Source: three-view drawing plus pictorial views. Frame: mm from the lowest corner of the part. A direction names the side the tool comes from. Coordinates: 2 decimals unless noted, no trailing zeros. Loops run counter-clockwise (first coordinate to the right, second up) from the corner with the lowest first, then second, coordinate; pieces in that order, holes last. Notation, with made-up numbers: (-29, -34.5) - (22, -34.5) arc R23 ccw to (22, -4.5) - close; hole circle Ø2 at (41, 61.25). An arc over 180 degrees is marked (long way). Return JSON: item names as keys, results as strings.
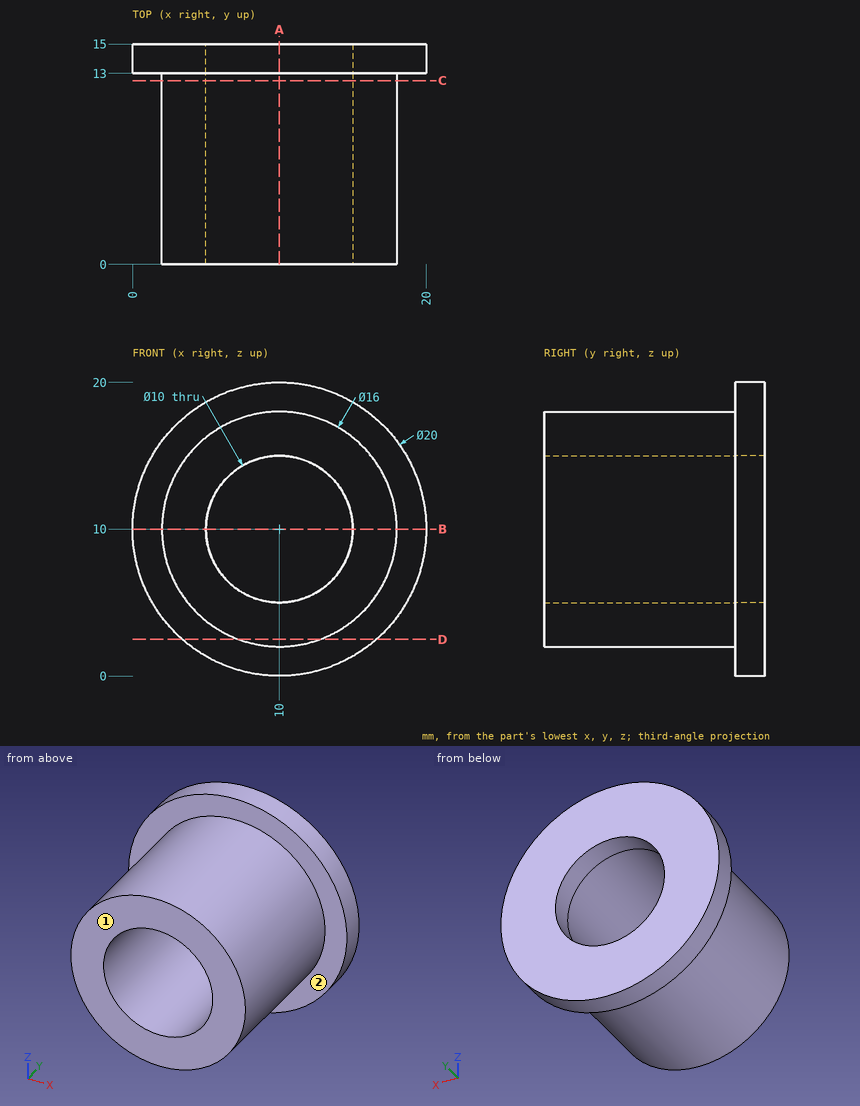
Item 1: Section query D-D, the plane z = 2.5. Return loops of the section in (x, y).
Worked out:
{"outline": "(3.39, 13) - (7.22, 13) - (7.22, 0) - (12.78, 0) - (12.78, 13) - (16.61, 13) - (16.61, 15) - (3.39, 15) - close"}
Item 2: First-contact query: pin 1 Ø6 at (y, z) = (1.5, 8) entering from -X; pin 2 Ø1 at (x, y) = (6.5, 13.5) entering from -Z; pin 3 Ø4 at (y, z) = (3, 4) entering from +X. Flat tips, straight axial feed; report the tip coordinate or a pass-through.
Worked out:
{"pin 1": "x = 2", "pin 2": "z = 0.46", "pin 3": "x = 16.93"}
Item 3: Section query A-A, the plane x = 10. Return loops of the section in (y, z), and give its area (3 significant figures).
Worked out:
{"outline": "(0, 2) - (13, 2) - (13, 0) - (15, 0) - (15, 5) - (0, 5) - close; (0, 15) - (15, 15) - (15, 20) - (13, 20) - (13, 18) - (0, 18) - close", "area": "98.0 mm^2"}
Item 4: Reachability of the marked faces 1 and 2 from +Z, -Z, +X, -X, +Y, -Y: full face, straight path, thin tool, end or side. Return the list, or none.
Worked out:
{"face 1": "+Z, -Z, +X, -X, -Y", "face 2": "-Y"}
Item 5: Ray query, probe 1 along Z at (x, y) = (10, 14.6); probe 2 along Z at (x, y) = (10, 6); probe 3 along Y at (x, z) = (17, 14.5). Return the intervals inside material, ascending. Write a range as from..to.
Worked out:
{"probe 1": "0..5, 15..20", "probe 2": "2..5, 15..18", "probe 3": "13..15"}
Item 6: Section query C-C, the plane y = 12.5. Return loops of the section in (x, z), and give its area (3 significant figures).
Worked out:
{"outline": "circle Ø16 at (10, 10); hole circle Ø10 at (10, 10)", "area": "123 mm^2"}
Item 7: Section query B-B, the plane z = 10. Return loops of the section in (x, y).
Worked out:
{"outline": "(0, 13) - (2, 13) - (2, 0) - (5, 0) - (5, 15) - (0, 15) - close; (15, 0) - (18, 0) - (18, 13) - (20, 13) - (20, 15) - (15, 15) - close"}
